Source: CAD feature listing. Evaluate the final solid. Frame: model axes, mm. A direction names the side the tool comes from. Coordinates: 2 decimals unless noted, no trailing zeros. Loops run counter-clockwise (first coordinate to the right, second up) from the corner with the lowest first, then second, coordinate; pieces in that order, holes last.
Item 1: Pin query (flat end, axial travel): pin 1 Ø4.5 at (x, y) = (12.7, 12.7) entering from +Z; pin 2 Ø3 at (y, z) = (26.5, 2) entering from -X. Return the tip coordinate at first contact, or that it passes through.
Item 2: Section query A-A, the plane x = 0. Return the cut outline in (y, z).
Item 3: Section query C-C, the plane z = 1.75. State how many separate pieces and enclosed holes the cut face has, then the cut area to 3 significant figures.
Item 4: Section query B-B, the plane x = 12.7. Return the cut outline in (y, z), then the cut area to 3 significant figures.
Item 5: Reachability of faces 5 (the flat face through (0, 20, 0)), 6 (the flat face through (22, 17.78, 3)), 7 (the flat face through (-17.78, 32, 3)) from +Z, -Z, +X, -X, +Y, -Y: full face, straight path, thin tool, end or side. Return the list, or none.
Item 6: Line query: probe 1 along Y at (x, z) = (12.7, 3.75); probe 2 along Y at (x, z) = (0, 2); probe 3 along Y at (x, z) = (-13.5, 1.25). Output: solid intervals per line, ascending.
Item 7: Section query D-D, the plane y = 12.7. Return the cut outline in (x, z).
Item 8: Pull-direction query (Y, two-part tool) for faces 1 (the cylindrical face through (24.45, 0.91, 3.13)), 2 (the flat face through (-22, 17.78, 3)), 3 (the flat face through (17.78, 32, 3)), 4 (the flat face through (-25.4, 9, 3)); classes: +Y half, -Y half, draft (parallel to the pull), parting line (faces both ways), or undercut.
```python
from build123d import *

# Parameters (mm, degrees)
SKETCH1_R           = 2.413
BOSS_EXTRUDE1_DEPTH = 6.35
FILLET1_R           = 3.175
FILLET3_R           = 2.54


with BuildPart() as part:
    # Sketch1 → Boss-Extrude1 (new body)
    with BuildSketch(Plane.XY):
        Polygon((-25.4, 0), (25.4, 0), (25.4, 17.78), (17.78, 17.78), (17.78, 45.72), (25.4, 45.72), (25.4, 50.8), (-25.4, 50.8), (-25.4, 45.72), (-17.78, 45.72), (-17.78, 17.78), (-25.4, 17.78), align=None)
        with Locations((-12.7, 12.7)):
            Circle(SKETCH1_R, mode=Mode.SUBTRACT)
        with Locations((12.7, 12.7)):
            Circle(SKETCH1_R, mode=Mode.SUBTRACT)
        with Locations((0, 25.4)):
            Circle(SKETCH1_R, mode=Mode.SUBTRACT)
        with Locations((-12.7, 38.1)):
            Circle(SKETCH1_R, mode=Mode.SUBTRACT)
        with Locations((12.7, 38.1)):
            Circle(SKETCH1_R, mode=Mode.SUBTRACT)
    extrude(amount=BOSS_EXTRUDE1_DEPTH)

    # Fillet1
    # the kernel refuses this fillet: 3.175 mm, written as the material it adds along each edge
    with BuildSketch(Plane(origin=(-17.78, 17.78, 0), x_dir=(0, 1, 0), z_dir=(0, 0, 1)), Plane(origin=(-17.78, 45.72, 0), x_dir=(-1, 0, 0), z_dir=(0, 0, 1)), Plane(origin=(17.78, 45.72, 0), x_dir=(0, -1, 0), z_dir=(0, 0, 1)), Plane(origin=(17.78, 17.78, 0), x_dir=(1, 0, 0), z_dir=(0, 0, 1))) as fillet1_piece_1:
        with BuildLine():
            CenterArc((FILLET1_R, FILLET1_R), FILLET1_R, 180, 90)
            Line((0, FILLET1_R), (0, 0))
            Line((0, 0), (FILLET1_R, 0))
        make_face()
    extrude(amount=6.35)
    # the kernel refuses this fillet: 3.175 mm, written as the material it takes off along each edge
    with BuildSketch(Plane(origin=(25.4, 0, -7.9375), x_dir=(-1, 0, 0), z_dir=(0, 0, 1)), Plane(origin=(-25.4, 45.72, -7.9375), x_dir=(0, 1, 0), z_dir=(0, 0, 1)), Plane(origin=(-25.4, 50.8, -7.9375), x_dir=(1, 0, 0), z_dir=(0, 0, 1)), Plane(origin=(25.4, 50.8, -7.9375), x_dir=(0, -1, 0), z_dir=(0, 0, 1)), Plane(origin=(25.4, 45.72, -7.9375), x_dir=(-1, 0, 0), z_dir=(0, 0, 1)), Plane(origin=(25.4, 17.78, -7.9375), x_dir=(0, -1, 0), z_dir=(0, 0, 1))) as fillet1_2_piece_1:
        with BuildLine():
            CenterArc((FILLET1_R, -FILLET1_R), FILLET1_R, 90, 90)
            Line((0, -FILLET1_R), (0, 0))
            Line((0, 0), (FILLET1_R, 0))
        make_face()
    extrude(amount=22.225, mode=Mode.SUBTRACT)
    with BuildSketch(Plane(origin=(-25.4, 0, -7.9375), x_dir=(1, 0, 0), z_dir=(0, 0, 1)), Plane(origin=(-25.4, 17.78, -7.9375), x_dir=(0, -1, 0), z_dir=(0, 0, 1))) as fillet1_2_piece_2:
        with BuildLine():
            CenterArc((FILLET1_R, FILLET1_R), FILLET1_R, 180, 90)
            Line((0, FILLET1_R), (0, 0))
            Line((0, 0), (FILLET1_R, 0))
        make_face()
    extrude(amount=22.225, mode=Mode.SUBTRACT)

    # Fillet3
    # the kernel refuses this fillet: 2.54 mm, written as the material it takes off along each edge
    with BuildSketch(Plane(origin=(-25.335851973, 48.26, 16.390208023), x_dir=(0.774595457226018, 0.6324570164404979, 0), z_dir=(0, 0, -1))) as fillet3_piece_1:
        with BuildLine():
            CenterArc((2.409649921, 1.967478618), FILLET3_R, 129.231849882, 179.999560802)
            ThreePointArc((0.803201559, 3.934944923), (-0.299592395, 2.110600119), (0, 0))
            ThreePointArc((0, 0), (2.008041601, -0.715651727), (4.016083202, 0))
        make_face()
    extrude(amount=26.430416045, mode=Mode.SUBTRACT)
    with BuildSketch(Plane(origin=(25.335851973, 48.26, 16.390208022), x_dir=(-0.774595458044749, -0.632457015437765, 0), z_dir=(0, 0, -1))) as fillet3_piece_2:
        with BuildLine():
            CenterArc((2.409649925, 1.967478616), FILLET3_R, 129.23184966, 179.999561099)
            ThreePointArc((0.80320157, 3.934944927), (-0.299592391, 2.110600124), (0, 0))
            ThreePointArc((0, 0), (2.008041604, -0.71565173), (4.016083209, 0))
        make_face()
    extrude(amount=26.430416044, mode=Mode.SUBTRACT)


solid = part.part
```
Verdict:
1. pin 1: passes through
1. pin 2: stops at x = -17.78
2. outline: (0, 0) - (22.99, 0) - (22.99, 6.35) - (0, 6.35) - close; (27.81, 0) - (50.8, 0) - (50.8, 6.35) - (27.81, 6.35) - close
3. separate pieces: 1
3. enclosed holes: 5
3. area: 2,050 mm2
4. outline: (0, 0) - (10.29, 0) - (10.29, 6.35) - (0, 6.35) - close; (15.11, 0) - (35.69, 0) - (35.69, 6.35) - (15.11, 6.35) - close; (40.51, 0) - (50.8, 0) - (50.8, 6.35) - (40.51, 6.35) - close
4. area: 261 mm2
5. face 5: -Z, +X, -X, +Y, -Y
5. face 6: +Z, -Z, +X
5. face 7: +Z, -Z, -X
6. probe 1: y = 0 to 10.29, 15.11 to 35.69, 40.51 to 50.8
6. probe 2: y = 0 to 22.99, 27.81 to 50.8
6. probe 3: y = 0 to 10.42, 14.98 to 35.82, 40.38 to 50.8
7. outline: (-25.4, 0) - (-15.11, 0) - (-15.11, 6.35) - (-25.4, 6.35) - close; (-10.29, 0) - (10.29, 0) - (10.29, 6.35) - (-10.29, 6.35) - close; (15.11, 0) - (25.4, 0) - (25.4, 6.35) - (15.11, 6.35) - close
8. face 1: -Y half
8. face 2: undercut
8. face 3: undercut
8. face 4: draft
